Geometry check sheet. Reference: the model listing, model coordinates, mm. Face numbers are marked on the shaded views. A direction names the side the tool comes from. Give positions to 0.01 mm unless a question says otherwise; leave off trailing zeros. Loops run counter-clockwise (first coordinate to the right, second up) from the corner with the lowest first, then second, coordinate; pieces in that order, holes last. Notation, with made-up numbers: (8.5, 58) -> (61.5, 58) arc R16 cw to (61.5, 71) -> close; hole circle Ø11 at (10, 49). An arc over 180 degrees is marked (long way). One line per item, written item: value. Start each with the question number.
(1) Gauge pin test, flat ends, axial feed: pin 1 Ø3.5 at (y, z) = (15.88, -154.82) entering from -X; pin 2 Ø6 at (x, y) = (0.5, 40.5) entering from +Z; pin 3 Ø8.5 at (x, z) = (133.35, -30.99) entering from +Y (3 decimals). Record the tip position at first contact, or that the pin passes through.
(2) Sectioned sample at A-A, the plane y = 25. Record the cut outline in (x, z), then the cut area to 3 significant figures.
(3) Scan lines: line 1 along Z through (x, y) = (133.35, 1.8); line 2 along Z through (x, y) = (120.5, 36.5); line 3 along X through (y, z) = (9, -63.5). Record each from-to range of solid material in increasing order. Write a range as from..to.
(4) Sectioned sample at C-C, the plane z = -150.5. Record the cut outline in (x, y) (3 decimals), then the cut area to 3 significant figures.
(5) Sectioned sample at B-B, the plane z = -71.5. Record the cut outline in (x, y) (3 decimals).
(6) Tool access check on the marked faces 1 and 2. Record the directions out of +Z, -Z, +X, -X, +Y, -Y that give a thin tool (end or side, any length) a straight path to the whole face; none if there is none.
from build123d import *

# Parameters (mm, degrees)
SKETCH1_R           = 3.175
BOSS_EXTRUDE1_DEPTH = 3.175
SKETCH2_W           = 6.35
SKETCH2_H           = 165.1
BOSS_EXTRUDE3_DEPTH = 6.35
SKETCH3_W           = 6.35
SKETCH3_H           = 12.7
BOSS_EXTRUDE4_DEPTH = 12.7
SKETCH4_W           = 6.35
SKETCH4_H           = 12.7
BOSS_EXTRUDE5_DEPTH = 25.4
FILLET1_R           = 6.35
FILLET3_R           = 6.35
CUT_EXTRUDE1_REACH  = 226.748
SKETCH6_R           = 1.5875


with BuildPart() as part:
    # Sketch1 → Boss-Extrude1 (new body)
    with BuildSketch(Plane(origin=(0, 0, 0), x_dir=(1, 0, 0), z_dir=(0, 1, 0))):
        with BuildLine():
            Line((-6.35, 161.169349013), (120.65, 161.169349013))
            Line((120.65, 161.169349013), (120.65, 142.119349013))
            ThreePointArc((120.65, 142.119349013), (122.509871939, 137.629220953), (127, 135.769349013))
            Line((127, 135.769349013), (133.35, 135.769349013))
            ThreePointArc((133.35, 135.769349013), (142.875, 126.244349013), (133.35, 116.719349013))
            Line((133.35, 116.719349013), (127, 116.719349013))
            ThreePointArc((127, 116.719349013), (122.509871939, 114.859477074), (120.65, 110.369349013))
            Line((120.65, 110.369349013), (120.65, 46.869349013))
            ThreePointArc((120.65, 46.869349013), (122.509871939, 42.379220953), (127, 40.519349013))
            Line((127, 40.519349013), (133.35, 40.519349013))
            ThreePointArc((133.35, 40.519349013), (142.875, 30.994349013), (133.35, 21.469349013))
            Line((133.35, 21.469349013), (127, 21.469349013))
            ThreePointArc((127, 21.469349013), (122.509871939, 19.609477074), (120.65, 15.119349013))
            Line((120.65, 15.119349013), (120.65, -3.930650987))
            Line((120.65, -3.930650987), (-6.35, -3.930650987))
            Line((-6.35, -3.930650987), (-6.35, 15.119349013))
            ThreePointArc((-6.35, 15.119349013), (-8.209871939, 19.609477074), (-12.7, 21.469349013))
            Line((-12.7, 21.469349013), (-19.05, 21.469349013))
            ThreePointArc((-19.05, 21.469349013), (-28.575, 30.994349013), (-19.05, 40.519349013))
            Line((-19.05, 40.519349013), (-12.7, 40.519349013))
            ThreePointArc((-12.7, 40.519349013), (-8.209871939, 42.379220953), (-6.35, 46.869349013))
            Line((-6.35, 46.869349013), (-6.35, 110.369349013))
            ThreePointArc((-6.35, 110.369349013), (-8.209871939, 114.859477074), (-12.7, 116.719349013))
            Line((-12.7, 116.719349013), (-19.05, 116.719349013))
            ThreePointArc((-19.05, 116.719349013), (-28.575, 126.244349013), (-19.05, 135.769349013))
            Line((-19.05, 135.769349013), (-12.7, 135.769349013))
            ThreePointArc((-12.7, 135.769349013), (-8.209871939, 137.629220953), (-6.35, 142.119349013))
            Line((-6.35, 142.119349013), (-6.35, 161.169349013))
        make_face()
        with Locations(Location((-19.05, 126.244349013, 0), (0, 0, 270))):
            Circle(SKETCH1_R, mode=Mode.SUBTRACT)
        with Locations(Location((-19.05, 30.994349013, 0), (0, 0, 270))):
            Circle(SKETCH1_R, mode=Mode.SUBTRACT)
        with Locations(Location((133.35, 30.994349013, 0), (0, 0, 270))):
            Circle(SKETCH1_R, mode=Mode.SUBTRACT)
        with Locations(Location((133.35, 126.244349013, 0), (0, 0, 270))):
            Circle(SKETCH1_R, mode=Mode.SUBTRACT)
        with BuildLine():
            Line((81.593842457, 148.469349013), (32.706157543, 148.469349013))
            ThreePointArc((32.706157543, 148.469349013), (27.157404819, 145.207041228), (27.30998728, 138.772134277))
            Line((27.30998728, 138.772134277), (51.753829737, 99.36530019))
            ThreePointArc((51.753829737, 99.36530019), (57.15, 96.362514927), (62.546170263, 99.36530019))
            Line((62.546170263, 99.36530019), (86.99001272, 138.772134277))
            ThreePointArc((86.99001272, 138.772134277), (87.142595181, 145.207041228), (81.593842457, 148.469349013))
        make_face(mode=Mode.SUBTRACT)
        with BuildLine():
            Line((107.95, 126.185693187), (107.95, 31.05300484))
            ThreePointArc((107.95, 31.05300484), (103.340232575, 24.946116059), (96.203829737, 27.705790103))
            Line((96.203829737, 27.705790103), (66.698688048, 75.272134277))
            ThreePointArc((66.698688048, 75.272134277), (65.744858311, 78.619349013), (66.698688048, 81.96656375))
            Line((66.698688048, 81.96656375), (96.203829737, 129.532907923))
            ThreePointArc((96.203829737, 129.532907923), (103.340232575, 132.292581968), (107.95, 126.185693187))
        make_face(mode=Mode.SUBTRACT)
        with BuildLine():
            Line((81.593842457, 8.769349013), (32.706157543, 8.769349013))
            ThreePointArc((32.706157543, 8.769349013), (27.157404819, 12.031656799), (27.30998728, 18.46656375))
            Line((27.30998728, 18.46656375), (51.753829737, 57.873397836))
            ThreePointArc((51.753829737, 57.873397836), (57.15, 60.876183099), (62.546170263, 57.873397836))
            Line((62.546170263, 57.873397836), (86.99001272, 18.46656375))
            ThreePointArc((86.99001272, 18.46656375), (87.142595181, 12.031656799), (81.593842457, 8.769349013))
        make_face(mode=Mode.SUBTRACT)
        with BuildLine():
            Line((6.35, 126.185693187), (6.35, 31.05300484))
            ThreePointArc((6.35, 31.05300484), (10.959767425, 24.946116059), (18.096170263, 27.705790103))
            Line((18.096170263, 27.705790103), (47.601311952, 75.272134277))
            ThreePointArc((47.601311952, 75.272134277), (48.555141689, 78.619349013), (47.601311952, 81.96656375))
            Line((47.601311952, 81.96656375), (18.096170263, 129.532907923))
            ThreePointArc((18.096170263, 129.532907923), (10.959767425, 132.292581968), (6.35, 126.185693187))
        make_face(mode=Mode.SUBTRACT)
    extrude(amount=BOSS_EXTRUDE1_DEPTH)

    # Sketch2 → Boss-Extrude3 (add)
    with BuildSketch(Plane(origin=(0, 3.175, 0), x_dir=(1, 0, 0), z_dir=(0, 1, 0))):
        with Locations((-3.175, 78.619349013)):
            Rectangle(SKETCH2_W, SKETCH2_H)
        with Locations((117.475, 78.619349013)):
            Rectangle(SKETCH2_W, SKETCH2_H)
    extrude(amount=BOSS_EXTRUDE3_DEPTH)

    # Sketch3 → Boss-Extrude4 (add)
    with BuildSketch(Plane(origin=(0, 9.525, 0), x_dir=(1, 0, 0), z_dir=(0, 1, 0))):
        with Locations((-3.175, 154.819349013)):
            Rectangle(SKETCH3_W, SKETCH3_H)
        with Locations((117.475, 154.819349013)):
            Rectangle(SKETCH3_W, SKETCH3_H)
        with Locations((117.475, 2.419349013)):
            Rectangle(SKETCH3_W, SKETCH3_H)
        with Locations((-3.175, 2.419349013)):
            Rectangle(SKETCH3_W, SKETCH3_H)
    extrude(amount=BOSS_EXTRUDE4_DEPTH)

    # Sketch4 → Boss-Extrude5 (add)
    with BuildSketch(Plane(origin=(0, 22.225, 0), x_dir=(1, 0, 0), z_dir=(0, 1, 0))):
        with Locations((-3.175, 154.819349013)):
            Rectangle(SKETCH4_W, SKETCH4_H)
        with Locations((117.475, 154.819349013)):
            Rectangle(SKETCH4_W, SKETCH4_H)
    extrude(amount=BOSS_EXTRUDE5_DEPTH)

    # Fillet1
    fillet1_edges = [part.edges().sort_by_distance(p)[0] for p in [
        (117.475, 22.225, -8.769349013),
        (117.475, 22.225, 3.930650987),
        (-3.175, 22.225, 3.930650987),
        (-3.175, 22.225, -8.769349013),
        (117.475, 47.625, -148.469349013),
        (117.475, 47.625, -161.169349013),
        (-3.175, 47.625, -148.469349013),
        (-3.175, 47.625, -161.169349013),
        (117.475, 9.525, -148.469349013),
        (117.475, 9.525, -8.769349013),
        (-3.175, 9.525, -8.769349013),
        (-3.175, 9.525, -148.469349013),
    ]]
    fillet(fillet1_edges, radius=FILLET1_R - 0.0001)  # a hair under: the kernel refuses the full size

    # Fillet3
    fillet3_edges = [part.edges().sort_by_distance(p)[0] for p in [
        (120.65, 3.175, -30.994349013),
        (120.65, 3.175, -126.244349013),
        (-6.35, 3.175, -30.994349013),
        (-6.35, 3.175, -126.244349013),
    ]]
    fillet(fillet3_edges, radius=FILLET3_R - 0.0001)  # a hair under: the kernel refuses the full size

    # Cut-Extrude1: up to this face of the body (flat: up to its plane)
    cut_extrude1_end = Plane(part.part.faces().sort_by_distance((120.65, 4.76245, -13.401031504))[0])
    # Sketch6 → Cut-Extrude1 (cut, up to the picked face)
    with BuildSketch(Plane.ZY.offset(6.35), mode=Mode.PRIVATE) as cut_extrude1_sk1:
        with Locations((-154.819349013, 41.275)):
            Circle(SKETCH6_R)
    cut_extrude1_tool1 = split(extrude(cut_extrude1_sk1.sketch, amount=-CUT_EXTRUDE1_REACH, mode=Mode.PRIVATE), bisect_by=cut_extrude1_end, keep=Keep.BOTH, mode=Mode.PRIVATE)
    # Sketch6 → Cut-Extrude1 (cut, up to the picked face)
    with BuildSketch(Plane.ZY.offset(6.35), mode=Mode.PRIVATE) as cut_extrude1_sk2:
        with Locations((-154.819349013, 15.875)):
            Circle(SKETCH6_R)
    cut_extrude1_tool2 = split(extrude(cut_extrude1_sk2.sketch, amount=-CUT_EXTRUDE1_REACH, mode=Mode.PRIVATE), bisect_by=cut_extrude1_end, keep=Keep.BOTH, mode=Mode.PRIVATE)
    # Sketch6 → Cut-Extrude1 (cut, up to the picked face)
    with BuildSketch(Plane.ZY.offset(6.35), mode=Mode.PRIVATE) as cut_extrude1_sk3:
        with Locations((-2.419349013, 15.875)):
            Circle(SKETCH6_R)
    cut_extrude1_tool3 = split(extrude(cut_extrude1_sk3.sketch, amount=-CUT_EXTRUDE1_REACH, mode=Mode.PRIVATE), bisect_by=cut_extrude1_end, keep=Keep.BOTH, mode=Mode.PRIVATE)
    add(cut_extrude1_tool1.solids().sort_by(Axis((-6.35, 41.275, -154.819349), (1, 0, 0)))[0], mode=Mode.SUBTRACT)
    add(cut_extrude1_tool2.solids().sort_by(Axis((-6.35, 15.875, -154.819349), (1, 0, 0)))[0], mode=Mode.SUBTRACT)
    add(cut_extrude1_tool3.solids().sort_by(Axis((-6.35, 15.875, -2.419349), (1, 0, 0)))[0], mode=Mode.SUBTRACT)


solid = part.part
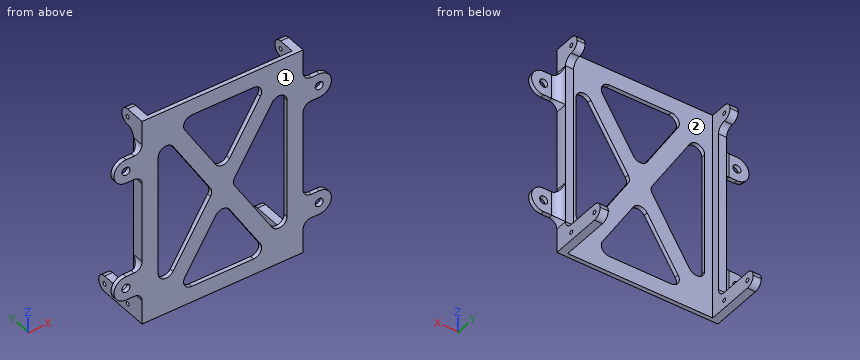
Calculated:
1. pin 1: stops at x = -6.35
1. pin 2: stops at z = -148.47
1. pin 3: stops at y = 3.175
2. outline: (-6.35, -161.17) -> (0, -161.17) -> (0, -148.47) -> (-6.35, -148.47) -> close; (114.3, -161.17) -> (120.65, -161.17) -> (120.65, -148.47) -> (114.3, -148.47) -> close
2. area: 161 mm2
3. line 1: z = -135.77..-129.42, -123.07..-116.72, -40.52..-34.17, -27.82..-21.47
3. line 2: z = -161.17..-148.47
3. line 3: x = -6.35..0, 114.3..120.65
4. outline: (-6.35, 0) -> (120.65, 0) -> (120.65, 45.93) -> (114.3, 45.93) -> (114.3, 3.175) -> (0, 3.175) -> (0, 45.93) -> (-6.35, 45.93) -> close
4. area: 946 mm2
5. outline: (-6.35, 0) -> (6.35, 0) -> (6.35, 3.175) -> (0, 3.175) -> (0, 9.525) -> (-6.35, 9.525) -> close; (45.261, 0) -> (69.039, 0) -> (69.039, 3.175) -> (45.261, 3.175) -> close; (107.95, 0) -> (120.65, 0) -> (120.65, 9.525) -> (114.3, 9.525) -> (114.3, 3.175) -> (107.95, 3.175) -> close
6. face 1: +Z, -Z, +X, -X, -Y
6. face 2: +Z, -Z, +Y
